Autodesk Inventor part; units mm, degrees
ref_plane "YZ Plane" through (0, 0, 0) normal (1, 0, 0) x (0, 1, 0)
ref_plane "XZ Plane" through (0, 0, 0) normal (0, 1, 0) x (-1, 0, 0)
ref_plane "XY Plane" through (0, 0, 0) normal (0, 0, 1) x (1, 0, 0)
sketch "Sketch1" plane through (0, 0, 0) normal (0, 1, 0) x (-1, 0, 0)
  line L0 (-4.0415, -7) -> (-8.0829, 0)
  line L1 (-8.0829, 0) -> (-4.0415, 7)
  line L2 (-4.0415, 7) -> (4.0415, 7)
  line L3 (4.0415, 7) -> (8.0829, 0)
  line L4 (8.0829, 0) -> (4.0415, -7)
  line L5 (4.0415, -7) -> (-4.0415, -7)
  circle A0 centre (0, 0) radius 5
  dimension "d0" = 14
  dimension "d1" = 10
extrude "Extrusion1" add sketch "Sketch1" along normal blind 2.5
thread "Thread1"
sketch "Sketch3" plane through (0, 0, 0) normal (1, 0, 0) x (0, 1, 0)
  line L0 (3.5, -5) -> (3.5, -9)
  line L1 (3.5, -9) -> (-1, -9)
  line L2 (2.5, -7) -> (2.5, 0)
  line L3 (0, -7) -> (2.5, -7)
  line L4 (0, 0) -> (10, 0) construction
  line L5 (-1, -9) -> (-1, -5)
  line L6 (-1, -5) -> (1, -8.5)
  line L7 (1, -8.5) -> (1.5, -8.5)
  line L8 (1.5, -8.5) -> (3.5, -5)
  line L9 (0, 0) -> (0, -7)
  dimension "d7" = 1
  dimension "d8" = 4
  dimension "d9" = 2
  dimension "d11" = 10
  dimension "d14" = 0.5
  dimension "d15" = 1
  dimension "d16" = 0.5
  dimension "d17" = 4
  dimension "d18" = 1
revolve "Revolution1" cut sketch "Sketch3" angle 360 about axis through (0, 0, 0) along (0, 1, 0) contours L0 L1 L5 L6 L9 L3 L7 L8 L2 | L2 L3 L8 | L3 L9 L6
chamfer "Chamfer1" distance 0.25 angle 45 6 edges at (-8.0829, 1.25, 0) (-4.0415, 1.25, -7) (4.0415, 1.25, -7) (8.0829, 1.25, 0) (4.0415, 1.25, 7) (-4.0415, 1.25, 7)
equation "\"d17\" = d8"
properties part number "4024-86" material "Brass"
For this review, take the finished solid that the model builds, in its own axes (mm). Give positions to 0.01 mm unless a question says otherwise; leave off trailing zeros. Order: outer loops, then holes, each group sorted by start corner. A loop starts at its lowest first (then second) coordinate and runs counter-clockwise, first axis right, second up. Notation, with made-up numbers: M 26,72.5 L 70,72.5 A32 ccw 70,100.5 Z; hole C -10,84 d7. An arc over 180 degrees is marked long. Answer in a Markdown table with one row per item. Add a question column.
(1) Wall thickness on probe 1 along Z at (x, y) = (0, 1.5); probe 2 along Z at (x, y) = (-3.75, 1.6); probe 3 along X at (y, z) = (2, 0.5): over which ranges is each line inside the solid? List them lowest first. Write a range as [from, to].
(2) Mouldability with a two-part tool opening along X and no side actions: class faces 1 (the face through (6.036, 1.235, -3.546)), 2 (the face through (5, 2.5, -2)), 3 (the face through (1.08, 1.23, 4.88)) as +X half, -X half, draft (parallel to the pull), parting line (faces both ways), or undercut.
(3) Consider section A-A on z = 0. State the section outline as (x, y) points, and give its area (3 significant figures).
(4) For pin 1 (1 mm diameter, centred on x = -6.5, y = 2, fed in from -Z), flat-tipped, find the tip position at first contact; note if it passes through.
(5) Consider section C-C on y = 1.1. State the section outline as (x, z) points, and give its area (3 significant figures).
(6) Consider section B-B on x = 0. State the section outline as (y, z) points, and give its area (3 significant figures).
Evaluation:
| question | item | result |
|---|---|---|
| 1 | probe 1 | z = [-7, -5], [5, 7] |
| 1 | probe 2 | z = [-7, -3.31], [3.31, 7] |
| 1 | probe 3 | x = [-7.61, -4.97], [4.97, 7.61] |
| 2 | face 1 | +X half |
| 2 | face 2 | draft |
| 2 | face 3 | undercut |
| 3 | outline | M -7.96,0.69 L -6.75,0 L -5,0 L -5,2.5 L -6.75,2.5 L -7.96,1.81 Z; M 5,0 L 6.75,0 L 7.96,0.69 L 7.96,1.81 L 6.75,2.5 L 5,2.5 Z |
| 3 | area | 13.1 mm^2 |
| 4 | pin 1 | stops at z = -3.61 |
| 5 | outline | M -7.96,-0.22 L -4.17,-6.78 L -3.79,-7 L 3.79,-7 L 4.17,-6.78 L 7.96,-0.22 L 7.96,0.22 L 4.17,6.78 L 3.79,7 L -3.79,7 L -4.17,6.78 L -7.96,0.22 Z; hole C 0,0 d10 |
| 5 | area | 91.0 mm^2 |
| 6 | outline | M 0,-6.75 L 0.14,-7 L 2.36,-7 L 2.5,-6.75 L 2.5,-5 L 0,-5 Z; M 0,5 L 2.5,5 L 2.5,6.75 L 2.36,7 L 0.14,7 L 0,6.75 Z |
| 6 | area | 9.93 mm^2 |
